Here's how the part is built. I have some questions about the finished solid (model axes, mm). A direction names the side the tool comes from. Coordinates: 2 decimals unless noted, no trailing zeros. Write each loop counter-clockwise with the first axis right and the second up, starting at its lowest first coordinate (ties: lowest second). Pieces come first, ordered by that corner, then holes. Notation, with made-up numbers: (89, 17.5) -> (122, 17.5) arc R30 ccw to (122, 51.5) -> close; hole circle Ø9 at (55, 38.5). An arc over 180 degrees is marked (long way). Put each result on its own line as item: value.
```python
from build123d import *
from build123d.topology import SkipClean

# Parameters (mm, degrees)
SKETCH_1_R               = 50
EXTRUDE_1_DEPTH          = 10
SKETCH_2_R               = 1.9999999999999927
CUT_EXTRUDE_1_DEPTH      = 72.4142842854285
PATTERN_CIRCULAR_1_COUNT = 8
SKETCH_6_R               = 30
EXTRUDE_4_DEPTH          = 10
EXTRUDE_START            = -10
EXTRUDE_5_DEPTH          = 10
SKETCH_8_R               = 35
EXTRUDE_6_DEPTH          = 10
SKETCH_9_R               = 25.200000000000003
CUT_EXTRUDE_2_DEPTH      = 10
SKETCH_10_R              = 35
SKETCH_10_R_2            = 25.20000000000001
EXTRUDE_7_DEPTH          = 7.5
SKETCH_11_R              = 35
SKETCH_11_R_2            = 1.2500000000000047
SKETCH_11_R_3            = 1.2500000000000013
SKETCH_11_R_4            = 12.000000000000005
EXTRUDE_8_DEPTH          = 7
SKETCH_12_R              = 30
SKETCH_12_R_2            = 17.85
EXTRUDE_9_DEPTH          = 35
EXTRUDE_START_2          = 7
SKETCH_16_R              = 34.099999999999994
SKETCH_16_R_2            = 32.59999999999999
EXTRUDE_12_DEPTH         = 7
EXTRUDE_START_3          = 1.7
SKETCH_17_R              = 35
SKETCH_17_R_2            = 34.099999999999994
EXTRUDE_13_DEPTH         = 1.7
CUT_EXTRUDE_3_DEPTH      = 39.00000000000001
PATTERN_CIRCULAR_2_COUNT = 2
PATTERN_CIRCULAR_2_ANGLE = 90.0000000000002
EXTRUDE_14_DEPTH         = 5
EXTRUDE_14_DEPTH_BACK    = 5
SKETCH_19_R              = 37.50000000000001
SKETCH_19_R_2            = 30
EXTRUDE_15_REACH         = 139.9
SKETCH_22_R              = 30
EXTRUDE_16_DEPTH         = 5
EXTRUDE_17_DEPTH         = 5


with BuildPart() as part:
    # 草图1 → 凸台-拉伸1 (new body)
    with BuildSketch(Plane(origin=(0, 0, 0), x_dir=(1, 0, 0), z_dir=(0, 1, 0))):
        with Locations(Location((0, 0, 0), (0, 0, 270))):
            Circle(SKETCH_1_R)
    extrude(amount=EXTRUDE_1_DEPTH)

    # 草图2 → 切除-拉伸1 (cut, through all)
    with BuildSketch(Plane(origin=(0, 10, 0), x_dir=(1, 0, 0), z_dir=(0, 1, 0))):
        with Locations(Location((0, -15.999999999999996, 0), (0, 0, 270))):
            Circle(SKETCH_2_R)
    cut_extrude_1 = extrude(amount=-CUT_EXTRUDE_1_DEPTH, mode=Mode.SUBTRACT)

    # 阵列(圆周)1: 切除-拉伸1 ×8 about axis
    pattern_circular_1_axis = Axis((1.404e-14, 0, 3e-17), (0, 1, 0))
    for i in range(1, PATTERN_CIRCULAR_1_COUNT):
        add(cut_extrude_1.rotate(pattern_circular_1_axis, i * 360 / PATTERN_CIRCULAR_1_COUNT), mode=Mode.SUBTRACT)

    # 草图6 → 凸台-拉伸4 (add)
    with BuildSketch(Plane(origin=(-20, 0, 0), x_dir=(0, 0, -1), z_dir=(1, 0, 0))):
        with Locations((-45.00000000000001, 48)):
            Circle(SKETCH_6_R)
        with BuildLine():
            Line((-66.57470511060487, 27.1545664619217), (-50, 10))
            Line((-50, 10), (20, 10))
            Line((20, 10), (-20.793603948134574, 65.72146693082246))
            ThreePointArc((-20.793603948134578, 65.72146693082246), (-16.48516279587097, 57.322234668898794), (-15.000000000000007, 48))
            ThreePointArc((-15.000000000000007, 47.99999999999999), (-33.75813968504649, 20.185964394588957), (-66.57470511060488, 27.154566461921696))
        make_face()
    extrude(amount=-EXTRUDE_4_DEPTH)

    # 草图7 → 凸台-拉伸5 (add)
    with BuildSketch(Plane.XZ.offset(EXTRUDE_START)):
        with BuildLine():
            Line((-20, 50.000000000000014), (-30, 50.000000000000014))
            Line((-30, 50.000000000000014), (-44.11764705882355, 23.52941176470589))
            ThreePointArc((-44.11764705882352, 23.529411764705895), (-25.724787771376317, 42.874646285627215), (3.06e-15, 50))
            Line((0, 50), (-20, 50.000000000000014))
        make_face()
    extrude(amount=EXTRUDE_5_DEPTH)

    # 草图8 → 凸台-拉伸6 (add)
    with BuildSketch(Plane.ZY.offset(30)):
        with Locations((45.00000000000001, 48)):
            Circle(SKETCH_8_R)
    extrude(amount=-EXTRUDE_6_DEPTH)

    # 草图9 → 切除-拉伸2 (cut)
    with BuildSketch(Plane.ZY.offset(30)):
        with Locations((45.00000000000001, 48)):
            Circle(SKETCH_9_R)
    extrude(amount=-CUT_EXTRUDE_2_DEPTH, mode=Mode.SUBTRACT)

    # 草图10 → 凸台-拉伸7 (add)
    with SkipClean():  # the faces are left unmerged after this step: merging them gives an invalid solid
        with BuildSketch(Plane(origin=(-20, 0, 0), x_dir=(0, 0, -1), z_dir=(1, 0, 0))):
            with Locations(Location((-45.00000000000001, 48, 0), (0, 0, 255.017807985))):
                Circle(SKETCH_10_R)
            with Locations(Location((-45.00000000000001, 48, 0), (0, 0, 180))):
                Circle(SKETCH_10_R_2, mode=Mode.SUBTRACT)
        extrude(amount=EXTRUDE_7_DEPTH)

    # 草图11 → 凸台-拉伸8 (add)
    with SkipClean():  # the faces are left unmerged after this step: merging them gives an invalid solid
        with BuildSketch(Plane(origin=(-12.5, 0, 0), x_dir=(0, 0, -1), z_dir=(1, 0, 0))):
            with Locations(Location((-45.00000000000001, 48, 0), (0, 0, 255.017807985))):
                Circle(SKETCH_11_R)
            with Locations((-45.00000000000001, 63)):
                Circle(SKETCH_11_R_2, mode=Mode.SUBTRACT)
            with Locations((-30.000000000000007, 48)):
                Circle(SKETCH_11_R_3, mode=Mode.SUBTRACT)
            with Locations((-60.00000000000001, 48)):
                Circle(SKETCH_11_R_2, mode=Mode.SUBTRACT)
            with Locations((-45.00000000000001, 33)):
                Circle(SKETCH_11_R_2, mode=Mode.SUBTRACT)
            with Locations((-45.00000000000001, 48)):
                Circle(SKETCH_11_R_4, mode=Mode.SUBTRACT)
        extrude(amount=EXTRUDE_8_DEPTH)

    # 草图12 → 凸台-拉伸9 (add)
    with SkipClean():  # the faces are left unmerged after this step: merging them gives an invalid solid
        with BuildSketch(Plane(origin=(-5.500000000000001, 0, 0), x_dir=(0, 0, -1), z_dir=(1, 0, 0))):
            with Locations((-45.00000000000001, 48)):
                Circle(SKETCH_12_R)
            with Locations((-45.00000000000001, 48)):
                Circle(SKETCH_12_R_2, mode=Mode.SUBTRACT)
        extrude(amount=EXTRUDE_9_DEPTH)

    # 草图16 → 凸台-拉伸12 (add)
    # profile 1 of 2: a face of its own
    with SkipClean():  # the faces are left unmerged after this step: merging them gives an invalid solid
        with BuildSketch(Plane.ZY.offset(30).offset(EXTRUDE_START_2)):
            with BuildLine():
                ThreePointArc((54.04815853046854, 14.18978220703822), (72.7640554365388, 26.689035082455778), (80, 47.99999999999999))
                ThreePointArc((80, 48), (46.58925584695761, 82.96389946577628), (10.144327665547948, 51.17523323762416))
                ThreePointArc((10.144327665547948, 51.17523323762416), (22.4503250761864, 21.2322552158324), (54.04815853046854, 14.18978220703822))
            make_face()
            with Locations((45.00000000000001, 48)):
                Circle(SKETCH_16_R, mode=Mode.SUBTRACT)
        # profile 2 of 2: a face of its own
        with BuildSketch(Plane.ZY.offset(30).offset(EXTRUDE_START_2)):
            with Locations((45.00000000000001, 48)):
                Circle(SKETCH_16_R)
            with Locations((45.00000000000001, 48)):
                Circle(SKETCH_16_R_2, mode=Mode.SUBTRACT)
        extrude(amount=-EXTRUDE_12_DEPTH)

    # 草图17 → 凸台-拉伸13 (add)
    with SkipClean():  # the faces are left unmerged after this step: merging them gives an invalid solid
        with BuildSketch(Plane.ZY.offset(37).offset(EXTRUDE_START_3)):
            with Locations((45.00000000000001, 48)):
                Circle(SKETCH_17_R)
            with Locations((45.00000000000001, 48)):
                Circle(SKETCH_17_R_2, mode=Mode.SUBTRACT)
        extrude(amount=-EXTRUDE_13_DEPTH)

    # 草图18 → 切除-拉伸3 (cut)
    with SkipClean():  # the faces are left unmerged after this step: merging them gives an invalid solid
        with BuildSketch(Plane.XY.offset(50)):
            with BuildLine():
                Line((-14.700000000000037, 55.50000000000001), (-14.700000000000031, 40.5))
                ThreePointArc((-14.700000000000031, 40.5), (-20.70000000000003, 34.5), (-26.700000000000035, 40.5))
                Line((-26.700000000000035, 40.5), (-26.70000000000004, 55.49999999999999))
                ThreePointArc((-26.70000000000004, 55.49999999999999), (-20.70000000000004, 61.5), (-14.700000000000037, 55.50000000000001))
            make_face()
        cut_extrude_3 = extrude(amount=CUT_EXTRUDE_3_DEPTH, mode=Mode.SUBTRACT)

    # 阵列(圆周)2: 切除-拉伸3 ×2 about axis
    with SkipClean():  # the faces are left unmerged after this step: merging them gives an invalid solid
        pattern_circular_2_axis = Axis((78.99494936611666, 48, 45.00000000000001), (-1, 0, 0))
        for i in range(1, PATTERN_CIRCULAR_2_COUNT):
            add(cut_extrude_3.rotate(pattern_circular_2_axis, i * PATTERN_CIRCULAR_2_ANGLE / (PATTERN_CIRCULAR_2_COUNT - 1)), mode=Mode.SUBTRACT)

    # 草图19 → 凸台-拉伸14 (add, two sides: drawn at the far end of the back side and taken through both)
    with SkipClean():  # the faces are left unmerged after this step: merging them gives an invalid solid
        with BuildSketch(Plane(origin=(-5.500000000000001, 0, 0), x_dir=(0, 0, -1), z_dir=(1, 0, 0)).offset(-EXTRUDE_14_DEPTH_BACK)):
            with Locations((-45.00000000000001, 48)):
                Circle(SKETCH_19_R)
            with Locations((-45.00000000000001, 48)):
                Circle(SKETCH_19_R_2, mode=Mode.SUBTRACT)
        extrude(amount=EXTRUDE_14_DEPTH + EXTRUDE_14_DEPTH_BACK)

    # 凸台-拉伸15: up to this face of the body (flat: up to its plane)
    extrude_15_end = Plane(part.part.faces().sort_by_distance((-0.5, 48, 81.439339828))[0])
    # 草图21 → 凸台-拉伸15 (add, up to the picked face)
    with BuildSketch(Plane(origin=(-20, 0, 0), x_dir=(0, 0, -1), z_dir=(1, 0, 0)), mode=Mode.PRIVATE) as extrude_15_sk1:
        with BuildLine():
            Line((-54.048158530468555, 14.189782207038219), (-50, 10.000000000000002))
            Line((-50, 10.000000000000002), (-25, 10))
            Line((-25, 10), (-20.789070824021746, 22.72489548120987))
            ThreePointArc((-20.78907082402175, 22.72489548120988), (-36.300032007942924, 14.098516891776221), (-54.048158530468555, 14.18978220703822))
        make_face()
    extrude_15_tool1 = split(extrude(extrude_15_sk1.sketch, amount=EXTRUDE_15_REACH, mode=Mode.PRIVATE), bisect_by=extrude_15_end, keep=Keep.BOTH, mode=Mode.PRIVATE)
    add(extrude_15_tool1.solids().sort_by(Axis((-20, 13.28361, 34.159805), (1, 0, 0)))[0])

    # 草图22 → 凸台-拉伸16 (add)
    with BuildSketch(Plane(origin=(29.500000000000004, 0, 0), x_dir=(0, 0, -1), z_dir=(1, 0, 0))):
        with Locations((-45.00000000000001, 48)):
            Circle(SKETCH_22_R)
        Polygon((-74.91061684419095, 47.99999999999995), (-45.00025054949128, 77.76927926767611), (-15.160260801057072, 47.92945668419983), (-45.07089861755983, 18.036484102537916), align=None, mode=Mode.SUBTRACT)
    extrude(amount=EXTRUDE_16_DEPTH)

    # 草图23 → 凸台-拉伸17 (add)
    with BuildSketch(Plane(origin=(29.500000000000004, 0, 0), x_dir=(0, 0, -1), z_dir=(1, 0, 0))):
        Polygon((-45.00025054949128, 77.76927926767611), (-47.004973093070014, 75.77401298888844), (-43.004973093070014, 75.77401298888844), align=None)
        Polygon((-72.91004844309327, 45.99113173137293), (-72.91004844309327, 49.99113173137294), (-74.91061684419095, 47.99999999999995), align=None)
        Polygon((-15.160260801057074, 47.92945668419983), (-17.160857181289597, 49.9300418570019), (-17.160857181289597, 45.930041857001896), align=None)
        Polygon((-43.06616767917176, 20.040031046019667), (-47.06616767917177, 20.040031046019667), (-45.07089861755983, 18.036484102537912), align=None)
    extrude(amount=EXTRUDE_17_DEPTH)


solid = part.part
```
Item 1: Imagine slicing it at B-B on z = -16. Write out the boundary of the cut face in (x, y).
Output:
outline: (-47.37, 0) -> (-2, 0) -> (-2, 10) -> (-20, 10) -> (-20, 15.46) -> (-30, 15.46) -> (-30, 10) -> (-47.37, 10) -> close; (2, 0) -> (47.37, 0) -> (47.37, 10) -> (2, 10) -> close
Item 2: For P1, Ø3, axis at x = 27, y = 53.5, coming from the +Z side; P2, Ø12, axis at x = -3.5, z = 51.5, coming from the +Y side; P3, Ø3, axis at x = 31.5, z = 45, coming from the +Y side, each with a flat end and sliding along its axis, tell me the tip position at first contact or that it passes through.
Output:
P1: stops at z = 74.73
P2: stops at y = 85.5
P3: stops at y = 78
Item 3: Imagine slicing it at A-A on x = 11. Write out the boundary of the cut face in (y, z) (3 decimals), then the cut area to 3 significant figures.
Output:
outline: (0, -48.775) -> (10, -48.775) -> (10, -13.289) -> (0, -13.289) -> close; (0, -9.338) -> (10, -9.338) -> (10, 9.338) -> (0, 9.338) -> close; (0, 13.289) -> (10, 13.289) -> (10, 48.775) -> (0, 48.775) -> close; circle Ø60 at (48, 45); hole circle Ø35.7 at (48, 45)
area: 2,720 mm²
Item 4: Please list where these lines run through material, in increasing order: line 1 along Y through (x, z) = (3.5, 35); line 2 along Y through (x, z) = (6, 17.5); line 3 along Y through (x, z) = (-9.25, 30). Write a range as from..to.
Output:
line 1: y = 0..10, 19.72..33.21, 62.79..76.28
line 2: y = 0..10, 36.01..59.99
line 3: y = 0..46.75, 49.25..82.37
Item 5: Imagine slicing it at C-C on x = 26. Write out the boundary of the cut face in (y, z), then the cut area to 3 significant figures.
Output:
outline: (0, -42.71) -> (10, -42.71) -> (10, 42.71) -> (0, 42.71) -> close; circle Ø60 at (48, 45); hole circle Ø35.7 at (48, 45)
area: 2,680 mm²
Item 6: Imagine slicing it at D-D on y = 38.5. State how many separate pieces and enclosed holes the cut face has, then the cut area to 3 significant figures.
Output:
separate pieces: 3
enclosed holes: 0
area: 1,880 mm²
Item 7: Which directions (+Z, -Z, +X, -X, +Y, -Y) give clear straight access to the entire face, cutting with the end or side of a thin tool? Please do faces 1 (the cylindrical face through (-20.8, 75.6, 31.5)), 2 (the flat face through (-36.96, 5.07, 36.95)), 3 (the cylindrical face through (-21.37, 32.67, 25)).
Output:
face 1: +Y
face 2: +Z, -X, -Y
face 3: -X
Item 8: If we mould it in two halves opening along Z, with no side actions, what happens to faces 4 (the flat face through (-30, 22, 9)), 5 (the flat face through (-15, 5, 50)), 6 (the cylindrical face through (-12.532, 5.07, -9.727))? For each: released by +Z, released by -Z, zero draft, split by the parting line, or undercut.
Output:
face 4: zero draft
face 5: released by +Z
face 6: undercut
